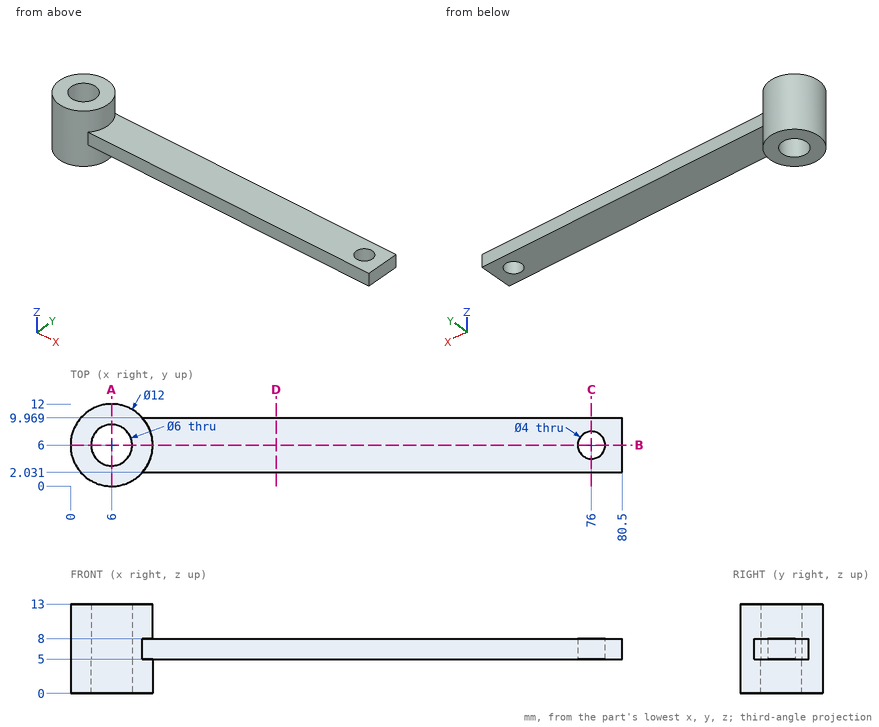
The figure shows three views and two pictorial views of one solid part (mm, origin at its lowest corner). Answer the questions. Give positions to 0.01 mm unless a question says otherwise; leave off trailing zeros. Write each loop counter-clockwise with the first axis right and the second up, starting at its lowest first coordinate (ties: lowest second). Pieces come first, ordered by that corner, then holes.
Q1. The part is cut by section C-C on x = 76. Give the vertices of the cut face in (y, z).
Answer:
outline: (2.03, 5) - (4, 5) - (4, 8) - (2.03, 8) - close; (8, 5) - (9.97, 5) - (9.97, 8) - (8, 8) - close
Q2. The part is cut by section D-D on x = 30. Give the vertices of the cut face in (y, z), and give its area (3 significant figures).
Answer:
outline: (2.03, 5) - (9.97, 5) - (9.97, 8) - (2.03, 8) - close
area: 23.8 mm2
Q3. Given pin 1 (2.5 mm diameter, centred on x = 52, z = 6.5, fed in from +Y); pin 2 (2.5 mm diameter, centred on x = 45, z = 6, fed in from -Y); pin 3 (6.5 mm diameter, centred on x = 33.5, y = 4.5, fed in from +Z), each flat-ended and moving along its own axis, determine where each tip first touches the part or whether it passes through.
Answer:
pin 1: stops at y = 9.97
pin 2: stops at y = 2.03
pin 3: stops at z = 8
Q4. Straight lines are drawn through the part: L1, parallel to Y at x = 6, z = 11.95; L2, parallel to Z at x = 57.5, y = 9.5; L3, parallel to X at y = 10.5, z = 5.75. For each, find the intervals that lie inside material, in ascending order.
Answer:
L1: y = 0 to 3, 9 to 12
L2: z = 5 to 8
L3: x = 2.03 to 9.97
Q5. The part is cut by section B-B on y = 6. Give the vertices of the cut face in (x, z).
Answer:
outline: (0, 0) - (3, 0) - (3, 13) - (0, 13) - close; (9, 0) - (12, 0) - (12, 5) - (74, 5) - (74, 8) - (12, 8) - (12, 13) - (9, 13) - close; (78, 5) - (80.5, 5) - (80.5, 8) - (78, 8) - close
Q6. The part is cut by section A-A on x = 6. Give the vertices of the cut face in (y, z), and give its area (3 significant figures).
Answer:
outline: (0, 0) - (3, 0) - (3, 13) - (0, 13) - close; (9, 0) - (12, 0) - (12, 13) - (9, 13) - close
area: 78.0 mm2
